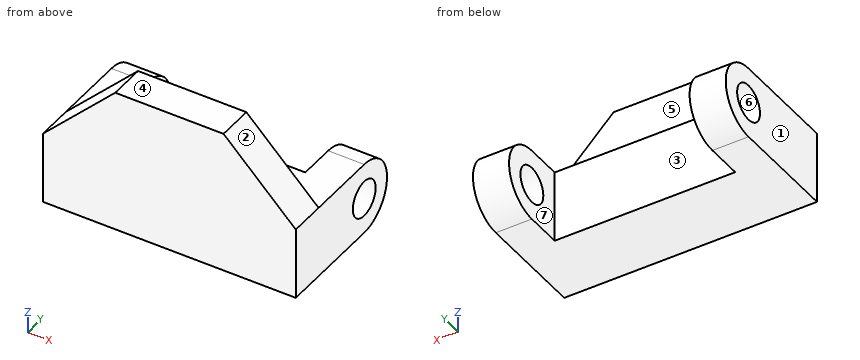
from build123d import *

# Parameters (mm, degrees)
BOSS_EXTRUDE1_DEPTH = 10
SKETCH1_3_W         = 50
SKETCH1_3_H         = 20
BOSS_EXTRUDE2_DEPTH = 20
SKETCH1_4_W         = 10
SKETCH1_4_H         = 20
BOSS_EXTRUDE3_DEPTH = 40
FILLET1_RADIUS      = 10
FILLET1_LENGTH      = 10
FILLET2_RADIUS      = 10
FILLET2_LENGTH      = 10
CUT_EXTRUDE1_REACH  = 76.833
SKETCH2_R           = 5
CUT_EXTRUDE2_START  = 60
SKETCH2_2_R         = 5
CUT_EXTRUDE2_DEPTH  = 70


with BuildPart() as part:
    # Sketch1 → Boss-Extrude1 (new body)
    with BuildSketch(Plane(origin=(0, 0, 0), x_dir=(1, 0, 0), z_dir=(0, 1, 0))):
        Polygon((20, -20), (0, 0), (70, 0), (50, -20), align=None)
    extrude(amount=BOSS_EXTRUDE1_DEPTH)

    # Sketch1<3> → Boss-Extrude2 (add)
    with BuildSketch(Plane(origin=(0, 0, 0), x_dir=(1, 0, 0), z_dir=(0, 1, 0))):
        with Locations((35, 10)):
            Rectangle(SKETCH1_3_W, SKETCH1_3_H)
    extrude(amount=BOSS_EXTRUDE2_DEPTH)

    # Sketch1<4> → Boss-Extrude3 (add)
    with BuildSketch(Plane(origin=(0, 0, 0), x_dir=(1, 0, 0), z_dir=(0, 1, 0))):
        with Locations((65, 10)):
            Rectangle(SKETCH1_4_W, SKETCH1_4_H)
        with Locations((5, 10)):
            Rectangle(SKETCH1_4_W, SKETCH1_4_H)
    extrude(amount=BOSS_EXTRUDE3_DEPTH)

    # Fillet1: full round fillet: the end face becomes a half cylinder, R = half its width
    fillet1_face = Plane((65, 40, -10), x_dir=(-1, 0, 0), z_dir=(0, 1, 0))  # on the end face: x along it, z out of the body
    fillet1_slab = fillet1_face.offset(-FILLET1_RADIUS / 2) * Box(FILLET1_LENGTH, 2 * FILLET1_RADIUS, FILLET1_RADIUS, mode=Mode.PRIVATE)  # the body's end, R deep
    fillet1_round = Plane((65, 30, -10), x_dir=(0, 1, 0), z_dir=(-1, 0, 0)) * Cylinder(FILLET1_RADIUS, FILLET1_LENGTH, mode=Mode.PRIVATE)  # its axis R under the face
    add(fillet1_slab - fillet1_round, mode=Mode.SUBTRACT)

    # Fillet2: full round fillet: the end face becomes a half cylinder, R = half its width
    fillet2_face = Plane((5, 40, -10), x_dir=(-1, 0, 0), z_dir=(0, 1, 0))  # on the end face: x along it, z out of the body
    fillet2_slab = fillet2_face.offset(-FILLET2_RADIUS / 2) * Box(FILLET2_LENGTH, 2 * FILLET2_RADIUS, FILLET2_RADIUS, mode=Mode.PRIVATE)  # the body's end, R deep
    fillet2_round = Plane((5, 30, -10), x_dir=(0, 1, 0), z_dir=(-1, 0, 0)) * Cylinder(FILLET2_RADIUS, FILLET2_LENGTH, mode=Mode.PRIVATE)  # its axis R under the face
    add(fillet2_slab - fillet2_round, mode=Mode.SUBTRACT)

    # Sketch2 → Cut-Extrude1 (cut, up to next)
    with BuildSketch(Plane.ZY.offset(-60), mode=Mode.PRIVATE) as cut_extrude1_sk1:
        with Locations((-10, 30)):
            Circle(SKETCH2_R)
    cut_extrude1_tool1 = extrude(cut_extrude1_sk1.sketch, amount=-CUT_EXTRUDE1_REACH, mode=Mode.PRIVATE) & part.part
    add(cut_extrude1_tool1.solids().sort_by_distance((60, 30, -10))[0], mode=Mode.SUBTRACT)

    # Sketch2<2> → Cut-Extrude2 (cut)
    with BuildSketch(Plane.ZY.offset(-60).offset(CUT_EXTRUDE2_START)):
        with Locations((-10, 30)):
            Circle(SKETCH2_2_R)
    extrude(amount=-CUT_EXTRUDE2_DEPTH, mode=Mode.SUBTRACT)


solid = part.part
Read the model definition and answer for the solid it produces. Units are mm, in the model's axes. Face numbers are marked on the shaded views. A direction names the side the tool comes from. Coordinates: 2 decimals unless noted, no trailing zeros. Loops run counter-clockwise (first coordinate to the right, second up) from the corner with the lowest first, then second, coordinate; pieces in that order, holes last. Notation, with made-up numbers: (-27, -9) -> (-6, -9) arc R27 cw to (-6, 27) -> close; hole circle Ø2 at (76.25, 49). An arc over 180 degrees is marked (long way). Write item = value, one per line. Start each with the question number.
1) The part is cut by section D-D, the plane x = 53.5. Determine the outline of the cut face in (y, z), plus the area to 3 significant figures.
2) The part is cut by section B-B, the plane x = 64.5. Determine the outline of the cut face in (y, z).
3) The mould has two halves that part along X. Classify the marked faces 1, 2, 3 and 4: pulls with the +X half, pulls with the -X half, needs draft (parallel to the pull), parting line crosses it, or undercut.
4) Given P1, Ø16, axis at y = 28.5, z = -6, coming from the -X side; P2, Ø4, axis at x = 16, y = 6, coming from the +Z side; P3, Ø16, axis at x = 29, z = 6.5, coming from the +Y side; P4, Ø2, axis at x = 10.5, y = 33.5, coming from the +Z side, each flat-ended and moving along its own axis, determine where each tip first touches the part or whether it passes through.
5) The part is cut by section A-A, the plane z = -10. Determine the outline of the cut face in (x, y).
6) For the marked faces 5, 6 and 7, determine the directions among +Z, -Z, +X, -X, +Y, -Y from which every point of the face is accessible in a straight line to the end or side of a thin tool.
7) The part is cut by section C-C, the plane y = 36. Determine the outline of the cut face in (x, z).
8) Find the intervals of material crossed by L1, parallel to Y at x = 7.5, z = -10; L2, parallel to Y at x = 42, z = -1.5; L3, parallel to Y at x = 29.5, z = 14, in increasing order. Write a range as from..to.
Result:
q1.outline = (0, -20) -> (20, -20) -> (20, 0) -> (10, 0) -> (10, 16.5) -> (0, 16.5) -> close
q1.area = 565 mm²
q2.outline = (0, -20) -> (30, -20) arc R10 ccw to (30, 0) -> (10, 0) -> (10, 5.5) -> (0, 5.5) -> close; hole circle Ø10 at (30, -10)
q3.face_1 = pulls with the -X half
q3.face_2 = pulls with the +X half
q3.face_3 = undercut
q3.face_4 = needs draft
q4.P1 = 0
q4.P2 = 18
q4.P3 = 20
q4.P4 = -0.35
q5.outline = (0, 0) -> (70, 0) -> (70, 25) -> (60, 25) -> (60, 20) -> (10, 20) -> (10, 25) -> (0, 25) -> close; (0, 35) -> (10, 35) -> (10, 40) -> (0, 40) -> close; (60, 35) -> (70, 35) -> (70, 40) -> (60, 40) -> close
q6.face_5 = +Z, +X, -X, +Y
q6.face_6 = +X, -X
q6.face_7 = +Z, -Z, +Y
q7.outline = (0, -18) -> (10, -18) -> (10, -2) -> (0, -2) -> close; (60, -18) -> (70, -18) -> (70, -2) -> (60, -2) -> close
q8.L1 = 0..25, 35..40
q8.L2 = 0..20
q8.L3 = 0..10
